Design review of the part built by this model. Coordinates are the model's own, in mm. A direction names the side the tool comes from. Coordinates: 2 decimals unless noted, no trailing zeros. Write each loop counter-clockwise with the first axis right and the second up, starting at its lowest first coordinate (ties: lowest second). Pieces come first, ordered by that corner, then holes. Notation, with made-up numbers: (40.5, 42) - (76.5, 42) arc R19 cw to (76.5, 73) - close; hole circle Ø11 at (-22, 45). An arc over 180 degrees is marked (long way). Use a Markdown table: item, result.
from build123d import *

# Parameters (mm, degrees)
SKETCH1_R           = 10
SKETCH1_R_2         = 5
BOSS_EXTRUDE1_DEPTH = 50
BOSS_EXTRUDE2_REACH = 46.087
SKETCH4_R           = 7.9
SKETCH6_R           = 4.7
BOSS_EXTRUDE3_DEPTH = 10
CHAMFER1_SIZE       = 1


with BuildPart() as part:
    # Sketch1 → Boss-Extrude1 (new body)
    with BuildSketch(Plane.XY):
        Circle(SKETCH1_R)
        Circle(SKETCH1_R_2, mode=Mode.SUBTRACT)
    extrude(amount=BOSS_EXTRUDE1_DEPTH)

    # Sketch4 → Boss-Extrude2 (add, up to next)
    with BuildSketch(Plane(origin=(0, 25, 32.738958199), x_dir=(-1, 0, 0), z_dir=(0, -0.939692621, -0.342020143)), mode=Mode.PRIVATE) as boss_extrude2_sk1:
        Circle(SKETCH4_R)
    boss_extrude2_tool1 = extrude(boss_extrude2_sk1.sketch, amount=BOSS_EXTRUDE2_REACH, mode=Mode.PRIVATE) - part.part
    add(boss_extrude2_tool1.solids().sort_by_distance((0, 25, 32.738958))[0])

    # Sketch6 → Boss-Extrude3 (add)
    with BuildSketch(Plane(origin=(0, 32.597653881, 11.86457572), x_dir=(1, 0, 0), z_dir=(0, 0.939692621, 0.342020143))):
        with Locations((0, -22.214053849)):
            Circle(SKETCH6_R)
    extrude(amount=BOSS_EXTRUDE3_DEPTH)

    # Chamfer1
    chamfer1_edges = [part.edges().sort_by_distance(p)[0] for p in [
        (-4.7, 34.396926208, 36.159159633),
    ]]
    chamfer(chamfer1_edges, length=CHAMFER1_SIZE)


solid = part.part
(1) Draft analysis for pull direction Y (two halves, no side actions). For faces 1 (the flat face through (-5, -2, 0)), 2 (the flat face through (-0.052, 34.415, 36.11)), 3 (the cylindrical face through (1.028, 18.191, 21.925)), state which applies: +Y half, -Y half, draft (parallel to the pull), parting line (faces both ways), or undercut.
Determined:
| item | result |
|---|---|
| face 1 | draft |
| face 2 | +Y half |
| face 3 | undercut |
(2) For pin 1 (1.5 mm diameter, centred on x = -1, y = 27.5, fed in from +Z); pin 2 (8 mm diameter, centred on y = -1.5, z = 41.5, fed in from +X); pin 3 (10 mm diameter, centred on y = 9, z = 11, fed in from +X); pin 4 (1.5 mm diameter, centred on x = -2, y = 20.5, fed in from -Z), all flat-tipped, find the tip position at first contact; note any pin that passes through.
Determined:
| item | result |
|---|---|
| pin 1 | z = 38.84 |
| pin 2 | x = 10 |
| pin 3 | x = 9.17 |
| pin 4 | z = 22.64 |
(3) Take a section at B-B on x = 0. Write out the cut boundary in (y, z).
Determined:
| item | result |
|---|---|
| outline | (-10, 0) - (-5, 0) - (-5, 50) - (-10, 50) - close; (5, 0) - (10, 0) - (10, 18.87) - (27.7, 25.32) - (26.61, 28.32) - (35.06, 31.4) - (35.66, 32.68) - (33.13, 39.64) - (31.85, 40.23) - (23.39, 37.16) - (22.3, 40.16) - (10, 35.69) - (10, 50) - (5, 50) - close |
(4) For L1, parallel to Y at x = -3, z = 17.5; L2, parallel to Y at x = -2.5, z = 10; L3, parallel to X at y = 1.5, z = 48, list the stretches that pass through material, from the lowest coordinate up. Write a range as from..to.
Determined:
| item | result |
|---|---|
| L1 | -9.54..-4, 4..9.54 |
| L2 | -9.68..-4.33, 4.33..9.68 |
| L3 | -9.89..-4.77, 4.77..9.89 |
(5) Machinability: for faces 4 (the flat face through (0.11, 23.24, 37.58)), 5 (the flat face through (-5, -2, 50)), which of the approach directions +Z, -Z, +X, -X, +Y, -Y give a long, thin tool a straight path to every point of the face, cutting with its end or side? Answer none if there is none.
Determined:
| item | result |
|---|---|
| face 4 | none |
| face 5 | +Z, +X, -X, +Y, -Y |
(6) Take a section at C-C on x = -7. Write out the cut boundary in (y, z).
Determined:
| item | result |
|---|---|
| outline | (-7.14, 0) - (7.14, 0) - (7.14, 22.34) - (26.25, 29.3) - (23.75, 36.18) - (7.14, 30.14) - (7.14, 50) - (-7.14, 50) - close |
(7) Take a section at A-A on y = 0. Write out the cut boundary in (x, z), and give its area (3 significant figures).
Determined:
| item | result |
|---|---|
| outline | (-10, 0) - (-5, 0) - (-5, 50) - (-10, 50) - close; (5, 0) - (10, 0) - (10, 50) - (5, 50) - close |
| area | 500 mm2 |
